from build123d import *

# Parameters (mm, degrees)
BOSS_EXTRUDE1_DEPTH = 110
SKETCH2_R           = 2
M_DRILL_DEPTH       = 20
SKETCH6_R           = 7.5
CUT_EXTRUDE2_DEPTH  = 10
SKETCH8_R           = 2.504958384
CUT_EXTRUDE3_DEPTH  = 10
CIRPATTERN1_COUNT   = 8


with BuildPart() as part:
    # Sketch1 → Boss-Extrude1 (new body)
    with BuildSketch(Plane(origin=(0, 0, 0), x_dir=(0, 0, -1), z_dir=(1, 0, 0))):
        Polygon((0, 0), (0, 19), (7.56469212, 19), (5, 13.5), (27.56469212, 13.5), (25, 8), (55, 8), (55, 0), align=None)
    extrude(amount=BOSS_EXTRUDE1_DEPTH)

    # Sketch2 → M$_DRILL (cut)
    with BuildSketch(Plane(origin=(0, 0, -55), x_dir=(-1, 0, 0), z_dir=(0, 0, -1))):
        with Locations((-20.948830341, 4.5)):
            Circle(SKETCH2_R)
        with Locations(Location((-89.051169659, 4.5, 0), (0, 0, 180))):
            Circle(SKETCH2_R)
    extrude(amount=-M_DRILL_DEPTH, mode=Mode.SUBTRACT)

    # Sketch6 → Cut-Extrude2 (cut)
    with BuildSketch(Plane(origin=(0, 8, 0), x_dir=(1, 0, 0), z_dir=(0, 1, 0))):
        with Locations(Location((54.829568948, 41.26029258, 0), (0, 0, 270))):
            Circle(SKETCH6_R)
    extrude(amount=-CUT_EXTRUDE2_DEPTH, mode=Mode.SUBTRACT)

    # Sketch8 → Cut-Extrude3 (cut)
    with BuildSketch(Plane(origin=(0, 8, 0), x_dir=(1, 0, 0), z_dir=(0, 1, 0))):
        with Locations(Location((39.829568948, 41.26029258, 0), (0, 0, 270))):
            Circle(SKETCH8_R)
    cut_extrude3 = extrude(amount=-CUT_EXTRUDE3_DEPTH, mode=Mode.SUBTRACT)

    # CirPattern1: Cut-Extrude3 ×8 about axis, 2 skipped
    cirpattern1_axis = Axis((54.829568948, 0, -41.26029258), (0, 1, 0))
    add([cut_extrude3.rotate(cirpattern1_axis, i * 360 / CIRPATTERN1_COUNT) for i in range(1, CIRPATTERN1_COUNT) if i not in (2, 6)], mode=Mode.SUBTRACT)


solid = part.part
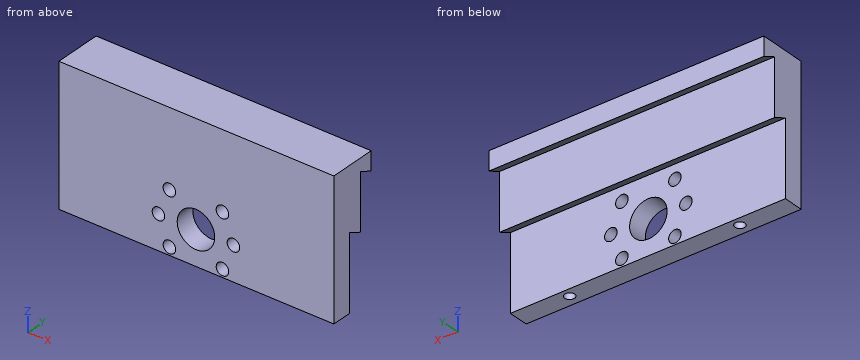
Design review of the part built by this model. Coordinates are the model's own, in mm. Round coordinates to 2 decimals unless told otherwise and drop trailing zeros. Write each loop counter-clockwise with the first axis right and the second up, starting at its lowest first coordinate (ties: lowest second). Pieces come first, ordered by that corner, then holes. Notation, with made-up numbers: (-7, -15) - (26, -15) arc R33 cw to (26, 19) - close; hole circle Ø9 at (19, 28). An arc over 180 degrees is marked (long way). Return JSON: item names as keys, results as strings. Group by question number.
Item 1: For probe 1 along Z at (x, y) = (44.5, 7.25); probe 2 along Y at (x, z) = (13, -30); probe 3 along Y at (x, z) = (34.5, -17), list the stretches that pass through material, from the lowest coordinate up. Write a range as [from, to].
Item 2: Insertion check: P1, Ø4, axis at x = 57.5, z = -11.5, coming from the +Y side; P2, Ø4, axis at x = 39.83, z = -41.26, coming from the +Y side; P3, Ø1, axis at x = 39, y = 13, coming from the +Z side; P4, Ø19.5, axis at x = 54.83, z = -41.26, coming from the +Y side. Each pin has a flat end and moves straight along its axis. Give the tip position at first contact, or say it passes through.
Item 3: We need section A-A on z = -42. Write out the cut boundary in (x, y).
Item 4: We need section C-C on y = 5.5. Write out the cut boundary in (x, z).
Item 5: We need section D-D on z = -9.5. Write out the cut boundary in (x, y).
Item 6: We need section B-B on x = 97. Write out the cut boundary in (y, z), and give its area (3 significant figures).
Model answer:
{
 "1": {"probe 1": "z = [-55, -54.36], [-49.38, -33.14], [-28.16, 0]", "probe 2": "y = [0, 8]", "probe 3": "y = [0, 13.5]"},
 "2": {"P1": "stops at y = 13.5", "P2": "passes through", "P3": "stops at z = 0", "P4": "stops at y = 8"},
 "3": {"outline": "(0, 0) - (37.44, 0) - (37.44, 8) - (0, 8) - close; (42.22, 0) - (47.37, 0) - (47.37, 8) - (42.22, 8) - close; (62.29, 0) - (67.44, 0) - (67.44, 8) - (62.29, 8) - close; (72.22, 0) - (110, 0) - (110, 8) - (72.22, 8) - close; hole circle Ø4 at (20.95, 4.5); hole circle Ø4 at (89.05, 4.5)"},
 "4": {"outline": "(0, -55) - (19.22, -55) - (19.22, -35) - (22.68, -35) - (22.68, -55) - (87.32, -55) - (87.32, -35) - (90.78, -35) - (90.78, -55) - (110, -55) - (110, 0) - (0, 0) - close; hole circle Ø5.01 at (39.83, -41.26); hole circle Ø5.01 at (44.22, -51.87); hole circle Ø5.01 at (44.22, -30.65); hole circle Ø15 at (54.83, -41.26); hole circle Ø5.01 at (65.44, -51.87); hole circle Ø5.01 at (65.44, -30.65); hole circle Ø5.01 at (69.83, -41.26)"},
 "5": {"outline": "(0, 0) - (110, 0) - (110, 13.5) - (0, 13.5) - close"},
 "6": {"outline": "(0, -55) - (8, -55) - (8, -25) - (13.5, -27.56) - (13.5, -5) - (19, -7.56) - (19, 0) - (0, 0) - close", "area": "619 mm²"}
}
